from build123d import *

# Parameters (mm, degrees)
SKETCH1_W           = 6.35
SKETCH1_H           = 19.05
SKETCH1_W_2         = 19.05
SKETCH1_R           = 2.413
BOSS_EXTRUDE1_DEPTH = 3.175
FILLET1_R           = 2.54
CUT_EXTRUDE1_REACH  = 5.175
SKETCH2_W           = 3.175
SKETCH2_H           = 6.35


with BuildPart() as part:
    # Sketch1 → Boss-Extrude1 (new body)
    with BuildSketch(Plane.XY):
        with Locations((-12.7, 0)):
            Rectangle(SKETCH1_W, SKETCH1_H)
        Rectangle(SKETCH1_W_2, SKETCH1_H)
        Circle(SKETCH1_R, mode=Mode.SUBTRACT)
        with Locations((12.7, 0)):
            Rectangle(SKETCH1_W, SKETCH1_H)
    extrude(amount=BOSS_EXTRUDE1_DEPTH)

    # Fillet1
    fillet1_edges = [part.edges().sort_by_distance(p)[0] for p in [
        (-15.875, -9.525, 1.5875),
        (-15.875, 9.525, 1.5875),
        (15.875, 9.525, 1.5875),
        (15.875, -9.525, 1.5875),
    ]]
    fillet(fillet1_edges, radius=FILLET1_R)

    # Sketch2 → Cut-Extrude1 (cut, up to next)
    with BuildSketch(Plane.XY.offset(3.175), mode=Mode.PRIVATE) as cut_extrude1_sk1:
        with Locations((7.9375, 0)):
            Rectangle(SKETCH2_W, SKETCH2_H)
    cut_extrude1_tool1 = extrude(cut_extrude1_sk1.sketch, amount=-CUT_EXTRUDE1_REACH, mode=Mode.PRIVATE) & part.part
    add(cut_extrude1_tool1.solids().sort_by_distance((7.9375, 0, 3.175))[0], mode=Mode.SUBTRACT)
    # Sketch2 → Cut-Extrude1 (cut, up to next)
    with BuildSketch(Plane.XY.offset(3.175), mode=Mode.PRIVATE) as cut_extrude1_sk2:
        with Locations((-7.9375, 0)):
            Rectangle(SKETCH2_W, SKETCH2_H)
    cut_extrude1_tool2 = extrude(cut_extrude1_sk2.sketch, amount=-CUT_EXTRUDE1_REACH, mode=Mode.PRIVATE) & part.part
    add(cut_extrude1_tool2.solids().sort_by_distance((-7.9375, 0, 3.175))[0], mode=Mode.SUBTRACT)


solid = part.part
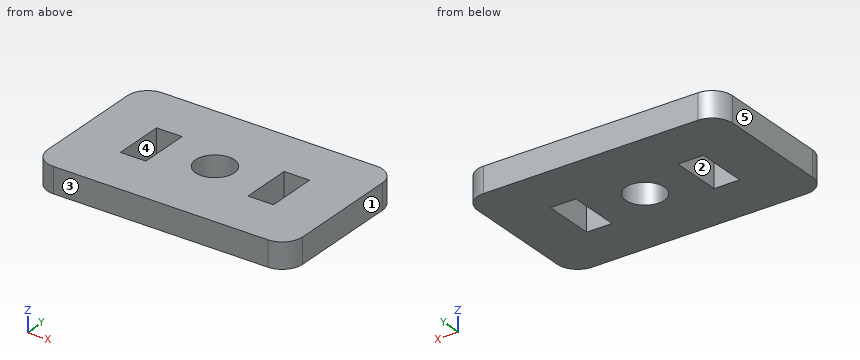
Model file for the job. Use its own axes, mm. Face numbers are marked on the shaded views. A direction names the side the tool comes from. Give positions to 0.01 mm unless a question says otherwise; leave off trailing zeros. Order: outer loops, then holes, each group sorted by start corner. A loop starts at its lowest first (then second) coordinate and runs counter-clockwise, first axis right, second up. Notation, with made-up numbers: M 12,31 L 71,31 A10 cw 71,35 Z; hole C -2,22 d6. An arc over 180 degrees is marked long. Put each result on its own line as item: value. Start each with the question number.
(1) Pull direction X, two halves, no side cores. Call the marked faces 1, 2 and 3: released by +X, released by -X, zero draft, split by the parting line, or undercut.
(2) Band-saw the part on A-A on x = 0. Give the cut face in (y, z) (3 decimals), then the cut area to 3 significant figures.
(3) Drill centre lines: L1, parallel to Y at x = 8.5, z = 1.9 (3 decimals); L2, parallel to X at y = -2, z = 0.3 (3 decimals); L3, parallel to Y at x = 0, z = 1.6 (3 decimals). Where is each one in solid material? Low to high. Write a range as [from, to].
(4) Band-saw the part on B-B on y = 0. Give the cut face in (x, z) (3 decimals).
(5) Band-saw the part on C-C on z = 0.3. Give the cut face in (x, y) (3 decimals).
(6) Band-saw the part on D-D on x = 7.5. Give the cut face in (y, z) (3 decimals), then the cut area to 3 significant figures.
(7) Tool access for the marked faces 4 and 5: list every direction of +Z, -Z, +X, -X, +Y, -Y with a clear straight run to the whole face (end or side of a thin tool).
Results below:
1. face 1: released by +X
1. face 2: undercut
1. face 3: zero draft
2. outline: M -9.525,0 L -2.413,0 L -2.413,3.175 L -9.525,3.175 Z; M 2.413,0 L 9.525,0 L 9.525,3.175 L 2.413,3.175 Z
2. area: 45.2 mm2
3. L1: y = [-9.525, -3.175], [3.175, 9.525]
3. L2: x = [-15.875, -9.525], [-6.35, -1.35], [1.35, 6.35], [9.525, 15.875]
3. L3: y = [-9.525, -2.413], [2.413, 9.525]
4. outline: M -15.875,0 L -9.525,0 L -9.525,3.175 L -15.875,3.175 Z; M -6.35,0 L -2.413,0 L -2.413,3.175 L -6.35,3.175 Z; M 2.413,0 L 6.35,0 L 6.35,3.175 L 2.413,3.175 Z; M 9.525,0 L 15.875,0 L 15.875,3.175 L 9.525,3.175 Z
5. outline: M -15.875,-6.985 A2.54 ccw -13.335,-9.525 L 13.335,-9.525 A2.54 ccw 15.875,-6.985 L 15.875,6.985 A2.54 ccw 13.335,9.525 L -13.335,9.525 A2.54 ccw -15.875,6.985 Z; hole M -9.525,-3.175 L -6.35,-3.175 L -6.35,3.175 L -9.525,3.175 Z; hole C 0,0 d4.826; hole M 6.35,-3.175 L 9.525,-3.175 L 9.525,3.175 L 6.35,3.175 Z
6. outline: M -9.525,0 L -3.175,0 L -3.175,3.175 L -9.525,3.175 Z; M 3.175,0 L 9.525,0 L 9.525,3.175 L 3.175,3.175 Z
6. area: 40.3 mm2
7. face 4: +Z, -Z
7. face 5: +Z, -Z, -X, +Y, -Y
